Here's the drawing with two shaded views (mm, measured from the low corner). I have some questions. A direction names the side the tool comes from. Give positions to 0.01 mm unless a question says otherwise; leave off trailing zeros. Write each loop counter-clockwise with the first axis right and the second up, starting at its lowest first coordinate (ties: lowest second). Pieces come first, ordered by that corner, then holes. Notation, with made-up numbers: (13.25, 32) - (55.25, 32) arc R14 cw to (55.25, 41) - close; hole circle Ø10 at (-2, 43). An arc over 180 degrees is marked (long way). Write item = value, one per line.
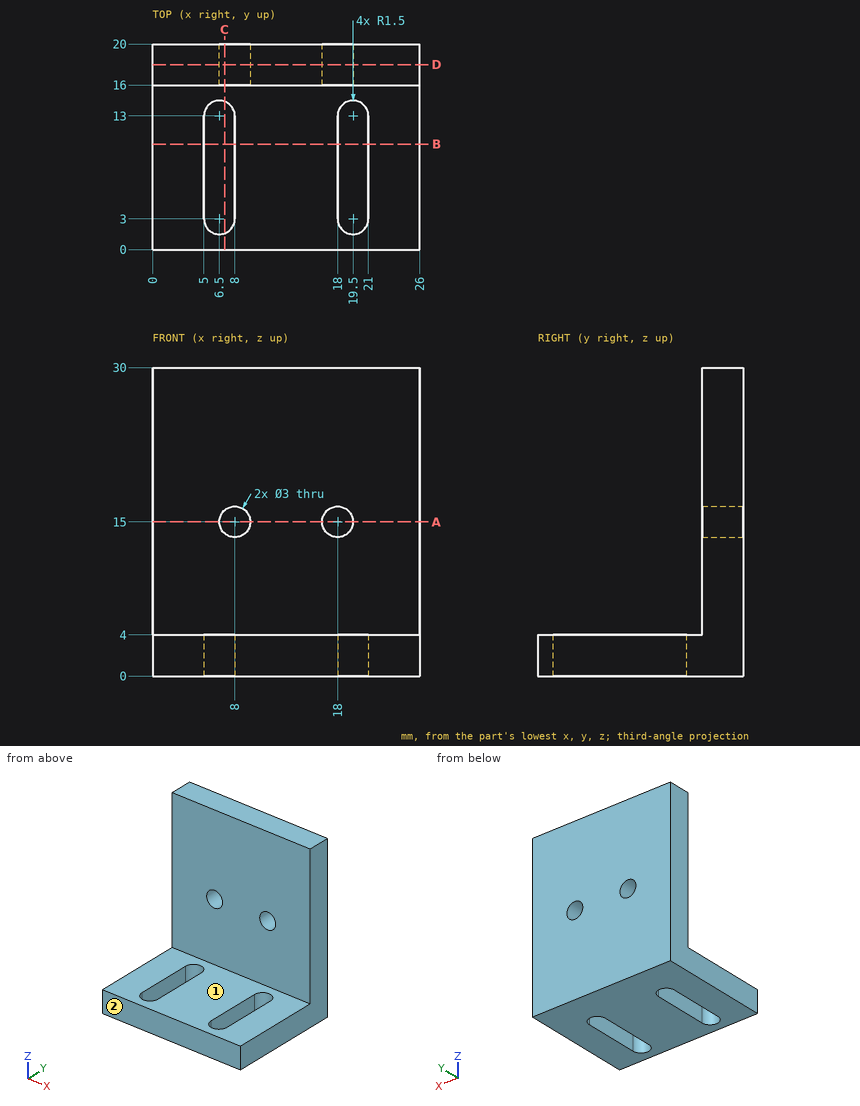
1. If we section it at B-B, the plane y = 10.25: Please give me the cut outline in (x, z).
Filled sheet:
outline = (0, 0) - (5, 0) - (5, 4) - (0, 4) - close; (8, 0) - (18, 0) - (18, 4) - (8, 4) - close; (21, 0) - (26, 0) - (26, 4) - (21, 4) - close
2. I need wall thicknesses on line 1 (X direction, y = 19.1, z = 15); line 2 (Z direction, x = 18, y = 18.2); line 3 (Y direction, x = 6, z = 25). Which ranges of each line are inside material? Lowest first, please.
Filled sheet:
line_1 = 0 to 6.5, 9.5 to 16.5, 19.5 to 26
line_2 = 0 to 13.5, 16.5 to 30
line_3 = 16 to 20
3. If we section it at D-D, the plane y = 18: Please give me the cut outline in (x, z).
Filled sheet:
outline = (0, 0) - (26, 0) - (26, 30) - (0, 30) - close; hole circle Ø3 at (8, 15); hole circle Ø3 at (18, 15)
4. Which directions (+Z, -Z, +X, -X, +Y, -Y) give clear straight access to the entire face, cutting with the end or side of a thin tool? Please do the marked faces 1 and 2.
Filled sheet:
face_1 = +Z, +X, -X, -Y
face_2 = +Z, -Z, +X, -X, -Y
5. If we section it at C-C, the plane x = 7: Please give me the cut outline in (y, z), and give its area (3 significant figures).
Filled sheet:
outline = (0, 0) - (1.59, 0) - (1.59, 4) - (0, 4) - close; (14.41, 0) - (20, 0) - (20, 13.88) - (16, 13.88) - (16, 4) - (14.41, 4) - close; (16, 16.12) - (20, 16.12) - (20, 30) - (16, 30) - close
area = 124 mm2
6. If we section it at A-A, the plane z = 15: Please give me the cut outline in (x, y), and give its area (3 significant figures).
Filled sheet:
outline = (0, 16) - (6.5, 16) - (6.5, 20) - (0, 20) - close; (9.5, 16) - (16.5, 16) - (16.5, 20) - (9.5, 20) - close; (19.5, 16) - (26, 16) - (26, 20) - (19.5, 20) - close
area = 80.0 mm2
7. For pin 1 (2.5 mm diameter, centred on x = 8, z = 15, fed in from +Y); pin 2 (8 mm diameter, centred on x = 21.5, z = 17.5, fed in from -Y); pin 3 (5 mm diameter, centred on x = 12.5, y = 11.5, fed in from +Z), each with a flat end and sliding along its axis, tell me the tip position at first contact or that it passes through.
Filled sheet:
pin_1 = through
pin_2 = 16
pin_3 = 4
